Geometry check sheet. Reference: the model listing, model coordinates, mm. Face numbers are marked on the shaded views. A direction names the side the tool comes from. Round coordinates to 2 decimals unless told otherwise and drop trailing zeros. Write each loop counter-clockwise with the first axis right and the second up, starting at its lowest first coordinate (ties: lowest second). Pieces come first, ordered by that corner, then holes. Notation, with made-up numbers: (16.25, -14.5) -> (27.25, -14.5) arc R24 cw to (27.25, -0.5) -> close; hole circle Ø6 at (81.25, 84). An arc over 180 degrees is marked (long way). Return JSON: item names as keys, results as strings. Group by question number.
Autodesk Inventor part; units mm, degrees
ref_plane "YZ Plane" through (0, 0, 0) normal (1, 0, 0) x (0, 1, 0)
ref_plane "XZ Plane" through (0, 0, 0) normal (0, 1, 0) x (-1, 0, 0)
ref_plane "XY Plane" through (0, 0, 0) normal (0, 0, 1) x (1, 0, 0)
sketch "Sketch1" plane through (0, 0, 0) normal (0, 1, 0) x (-1, 0, 0)
  line L0 (0, 0) -> (56, 0)
  line L1 (56, 0) -> (56, -85)
  line L2 (56, -85) -> (0, -85)
  line L3 (0, -85) -> (0, 0)
  line L4 (61, -90) -> (61, 5)
  line L5 (61, 5) -> (-5, 5)
  line L6 (-5, 5) -> (-5, -90)
  line L7 (61, -85) -> (-5, -85)
  dimension "d0" = 56
  dimension "d1" = 85
  dimension "d2" = 5
  dimension "d50" = 90
extrude "Extrusion1" add sketch "Sketch1" along normal blind 1
sketch "Sketch2" plane through (0, 1, 0) normal (0, 1, 0) x (1, 0, 0)
  line L0 (-61, -5) -> (5, -5)
  line L1 (-61, 85) -> (-61, -5)
  line L2 (-61, -5) -> (5, -5)
  line L3 (5, -5) -> (5, 85)
  line L4 (5, 85) -> (-61, 85)
  line L5 (-62, 86) -> (6, 86)
  line L6 (6, 86) -> (6, -6)
  line L7 (6, -6) -> (-62, -6)
  line L8 (-62, -6) -> (-62, 86)
  point P0 (0, 0)
  dimension "d41" = 1
sketch "Sketch4" plane through (0, 1, 0) normal (0, 1, 0) x (1, 0, 0)
  line L0 (0, 0) -> (-56, 0)
  line L1 (-56, 0) -> (-56, 85)
  line L2 (-56, 85) -> (0, 85)
  line L3 (0, 85) -> (0, 0)
  circle A0 centre (-3.5, 3.5) radius 1.375
  circle A1 centre (-52.5, 3.5) radius 1.375
  circle A2 centre (-52.5, 61.5) radius 1.375
  circle A3 centre (-3.5, 61.5) radius 1.375
  circle A4 centre (-52.5, 3.5) radius 3.1
  circle A5 centre (-52.5, 61.5) radius 3.1
  circle A6 centre (-3.5, 3.5) radius 3.1
  circle A7 centre (-3.5, 61.5) radius 3.1
  dimension "d14" = 56
  dimension "d15" = 85
  dimension "d16" = 2.75
  dimension "d17" = 2.75
  dimension "d18" = 2.75
  dimension "d19" = 2.75
  dimension "d20" = 49
  dimension "d21" = 58
  dimension "d22" = 58
  dimension "d23" = 49
  dimension "d24" = 6.2
  dimension "d25" = 6.2
  dimension "d26" = 6.2
  dimension "d27" = 6.2
  dimension "d28" = 3.5
  dimension "d29" = 3.5
  dimension "d30" = 3.5
  dimension "d31" = 3.5
  dimension "d32" = 3.5
hole "Hole1" at (-52.5, 1, -61.5) at (-52.5, 1, -3.5) at (-3.5, 1, -3.5) at (-3.5, 1, -61.5) direction (0, -1, 0) diameter 2.75 end through all
extrude "Extrusion4" add sketch "Sketch2" along normal blind 20 and the other way blind 1
sketch "Sketch5" plane through (6, 21, -86) normal (0, 0, -1) x (-1, 0, 0)
  line L0 (67, -20) -> (1, -20)
  line L1 (68, 0) -> (0, 0)
  line L2 (3, -20) -> (65, -20)
  line L3 (65, -20) -> (65, 0)
  line L4 (65, 0) -> (3, 0)
  line L5 (3, 0) -> (3, -20)
  line L6 (67, 0) -> (67, -20)
  line L7 (1, 0) -> (1, -20)
  point P0 (6, -21)
  dimension "d46" = 2
  dimension "d47" = 2
extrude "Extrusion5" cut sketch "Sketch5" against normal blind 2 contours L0 L5 L1 L3
sketch "Sketch6" plane through (6, 0, -86) normal (1, 0, 0) x (0, 0, -1)
  line L0 (0, 21) -> (0, 0)
  line L1 (-92, 21) -> (0, 21)
  line L2 (-92, 21) -> (-92, 0)
  line L3 (0, 0) -> (-92, 0)
  point P0 (-86, 0)
extrude "Extrusion6" add sketch "Sketch6" along normal blind 1.5
sketch "Sketch7" plane through (-62, 0, 6) normal (-1, 0, 0) x (0, 0, 1)
  line L0 (0, 21) -> (0, 0)
  line L1 (-92, 21) -> (0, 21)
  line L2 (-92, 0) -> (-92, 21)
  line L3 (0, 0) -> (-92, 0)
  point P0 (-6, 0)
extrude "Extrusion7" add sketch "Sketch7" along normal blind 1.5
sketch "Sketch8" plane through (0, 21, 0) normal (0, 1, 0) x (1, 0, 0)
  line L0 (7.5, -6) -> (-63.5, -6)
  line L1 (7.5, 86) -> (7.5, -6)
  line L2 (-63.5, -6) -> (-63.5, 86)
  line L3 (-59, 86) -> (3, 86)
  line L4 (-59, 86) -> (-63.5, 86)
  line L5 (3, 86) -> (7.5, 86)
  point P0 (0, 0)
  dimension "d55" = 92
  dimension "d56" = 71
sketch "Sketch9" plane through (-61, 1, 5) normal (1, 0, 0) x (0, 0, -1)
  line L0 (0, 0) -> (0, 20)
  line L1 (90, 20) -> (90, 0)
  line L2 (0, 20) -> (90, 20)
  line L3 (30, 16.25) -> (60, 16.25)
  line L4 (60, 16.25) -> (60, 14.75)
  line L5 (60, 14.75) -> (30, 14.75)
  line L6 (30, 14.75) -> (30, 16.25)
  point P0 (5, -1)
  point P1 (0, 16)
  point P2 (90, 15)
  dimension "d62" = 3.75
  dimension "d63" = 1.5
  dimension "d64" = 30
  dimension "d65" = 30
  dimension "d66" = 30
extrude "Extrusion8" cut sketch "Sketch9" against normal blind 1.5
ref_plane "Work Plane2" through (-28, 0, -86) normal (1, 0, 0) x (0, 0, -1)
mirror "Mirror1" about plane through (-28, 0, -86) normal (1, 0, 0) of "Extrusion8"
sketch "Sketch10" plane through (7.5, 0, -86) normal (1, 0, 0) x (0, 0, -1)
  line L0 (-91, 21) -> (-1, 21)
  line L1 (-85, 0.9618) -> (-67, 0.9618)
  line L2 (-67, 0.9618) -> (-67, 21)
  line L3 (-67, 21) -> (-85, 21)
  line L4 (-85, 21) -> (-85, 0.9618)
  line L5 (-92, 21) -> (-92, 0)
  point P0 (-86, 0)
  point P1 (-76, 0.9618)
  dimension "d67" = 7
  dimension "d68" = 18
  dimension "d69" = 16
  dimension "d72" = 25
extrude "Extrusion9" cut sketch "Sketch10" against normal blind 3
equation "\"d22\" = d21"
equation "\"d23\" = d20"
properties part number "bottom2"
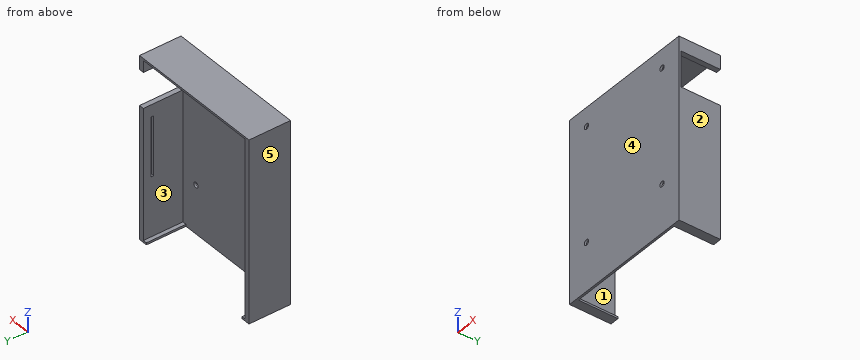
1) Sectioned sample at D-D on z = -35.5. Enter the section's corners in (x, y).
2) Mould release check, pull along X, two halves, no side actions. Record for the marked faces 3, 4 and 5: +X half, -X half, draft (parallel to the pull), parting line (faces both ways), or undercut.
3) Material ranges on probe 1 along Z at (x, y) = (-52.5, 0.8) (3 decimals); probe 2 along X at (y, z) = (0.45, -3.5) (3 decimals); probe 3 along X at (y, z) = (10.5, -75), recorded low to high. Write a range as [from, to].
4) Sectioned sample at C-C on y = 5.75. Enter the section's corners in (x, z).
5) Go/stop test with a flat-tipped pin: P1, Ø2, axis at x = -54.5, z = -9, coming from the +Y side. Record where the tip stops, or that it passes through.
6) Sectioned sample at A-A on x = -52.5. Enter the section's corners in (y, z) (3 decimals), and give its area (4 significant figures).
7) Sectioned sample at B-B on z = -3.5. Enter the section's corners in (x, y) (3 decimals), and give its area (3 significant figures).
8) Tool access check on the marked faces 1 and 2. Record the directions out of +Z, -Z, +X, -X, +Y, -Y that give a thin tool (end or side, any length) a straight path to the whole face; none if there is none.
Evaluation:
{
 "1": {"outline": "(-63.5, 0) -> (7.5, 0) -> (7.5, 21) -> (5, 21) -> (5, 17.25) -> (6.5, 17.25) -> (6.5, 15.75) -> (5, 15.75) -> (5, 1) -> (-61, 1) -> (-61, 15.75) -> (-62.5, 15.75) -> (-62.5, 17.25) -> (-61, 17.25) -> (-61, 21) -> (-63.5, 21) -> close"},
 "2": {"face 3": "undercut", "face 4": "draft", "face 5": "-X half"},
 "3": {"probe 1": "z = [-86, -62.875], [-60.125, -4.875], [-2.125, 6]", "probe 2": "x = [-63.5, -53.875], [-51.125, -4.875], [-2.125, 7.5]", "probe 3": "x = [-63.5, -61], [5, 7.5]"},
 "4": {"outline": "(-63.5, -86) -> (-59, -86) -> (-59, -85) -> (-61, -85) -> (-61, 5) -> (5, 5) -> (5, -1) -> (7.5, -1) -> (7.5, 6) -> (-63.5, 6) -> close; (3, -86) -> (7.5, -86) -> (7.5, -19) -> (5, -19) -> (5, -85) -> (3, -85) -> close"},
 "5": {"P1": "stops at y = 1"},
 "6": {"outline": "(0, -86) -> (1, -86) -> (1, -62.875) -> (0, -62.875) -> close; (0, -60.125) -> (1, -60.125) -> (1, -4.875) -> (0, -4.875) -> close; (0, -2.125) -> (1, -2.125) -> (1, 5) -> (21, 5) -> (21, 6) -> (0, 6) -> close", "area": "106.5 mm2"},
 "7": {"outline": "(-63.5, 0) -> (-53.875, 0) -> (-53.875, 1) -> (-61, 1) -> (-61, 21) -> (-63.5, 21) -> close; (-51.125, 0) -> (-4.875, 0) -> (-4.875, 1) -> (-51.125, 1) -> close; (-2.125, 0) -> (7.5, 0) -> (7.5, 0.962) -> (4.5, 0.962) -> (4.5, 1) -> (-2.125, 1) -> close", "area": "115 mm2"},
 "8": {"face 1": "+Y", "face 2": "+Z, -Z, +X, +Y, -Y"}
}
